Can you work these out from the model? Positions are in its coordinate system, mm. Face numbers are marked on the shaded views. A direction names the side the tool comes from. Give positions to 0.01 mm unless a question says otherwise; leave off trailing zeros. Order: outer loops, then holes, each group sorted by start corner. A loop starts at its lowest first (then second) coordinate and runs counter-clockwise, first axis right, second up.
Item 1: I want a section at D-D, the plane x = 25. Write out the boundary of the cut face in (y, z), then the cut area to 3 significant figures.
Item 2: If I drill on line 1 along X through (y, z) = (-4.25, -3.88); line 2 along Z through (x, y) = (25, -4.5); line 3 along Y through (x, z) = (10, 1.15), over which ranges is the centre line in solid material (lowest first)?
Item 3: I want a section at B-B, the plane y = -8. Write out the boundary of the cut face in (x, z), then the cut area to 3 significant figures.
Item 4: If we mould it in two halves opening along Z, with no side actions, what happens to the marked faces 1, 2 and 3? For each: +Z half, -Z half, draft (parallel to the pull), parting line (faces both ways), or undercut.
Item 5: I want a section at C-C, the plane z = -3.88. Write out the boundary of the cut face in (x, y), then the cut area to 3 significant figures.
Item 6: Which directions (+Z, -Z, +X, -X, +Y, -Y) give clear straight access to the entire face, cutting with the end or side of a thin tool? Please do the marked faces 4 and 5.
Item 7: I want a section at A-A, the plane x = 12. Write out the boundary of the cut face in (y, z).
Item 8: I'm going to push flat-ended pins straight in: pin 1 Ø1 at (y, z) = (-14, -4) entering from -X; pin 2 Ø2.5 at (x, z) = (24, -3) entering from +Y; pin 3 Ø3 at (x, y) = (10, -8) entering from -Z; pin 4 Ø1 at (x, y) = (3.5, -5.5) entering from -Z. Where does each tip first touch, or does it pass through?
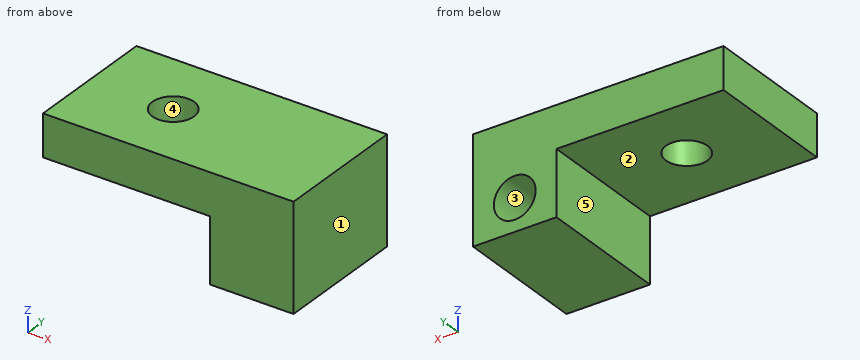
Autodesk Inventor part; units mm, degrees
ref_plane "YZ Plane" through (0, 0, 0) normal (1, 0, 0) x (0, 1, 0)
ref_plane "XZ Plane" through (0, 0, 0) normal (0, 1, 0) x (-1, 0, 0)
ref_plane "XY Plane" through (0, 0, 0) normal (0, 0, 1) x (1, 0, 0)
sketch "Sketch1" plane through (0, 0, 0) normal (0, 0, 1) x (1, 0, 0)
  line L0 (0, 0) -> (20, 0)
  line L1 (20, 0) -> (20, -16)
  line L2 (20, -16) -> (0, -16)
  line L3 (0, -16) -> (0, 0)
  circle A0 centre (10, -8) radius 2.5
  dimension "d0" = 20
  dimension "d1" = 16
  dimension "d2" = 8
  dimension "d3" = 10
  dimension "d4" = 5
extrude "Extrusion1" add sketch "Sketch1" along normal blind 5
sketch "Sketch2" plane through (0, 0, 0) normal (0, 1, 0) x (1, 0, 0)
  line L0 (20, 0) -> (20, -5)
  line L1 (20, 0) -> (30, 0)
  line L2 (30, 0) -> (30, 7.76)
  line L3 (30, 7.76) -> (20, 7.76)
  line L4 (20, 7.76) -> (20, 0)
  line L5 (20, -5) -> (30, -5)
  line L6 (30, -5) -> (30, 0)
  line L7 (30, 0) -> (20, 0)
  line L8 (20, 0) -> (20, -5)
  circle A0 centre (25, 3.88) radius 2.5
  point P0 (0, 0)
  dimension "d7" = 10
  dimension "d8" = 7.76
  dimension "d9" = 5
extrude "Extrusion2" add sketch "Sketch2" against normal blind 16
sketch "Sketch3" plane through (0, -16, 0) normal (0, -1, 0) x (1, 0, 0)
  line L0 (30, -7.76) -> (30, 5)
  line L1 (0, 0) -> (20, 0)
  line L2 (30, -7.76) -> (20, -7.76)
  line L3 (20, -7.76) -> (20, 0)
  line L4 (20, 0) -> (30, 0)
  line L5 (30, 0) -> (30, -7.76)
extrude "Extrusion3" add sketch "Sketch3" against normal blind 9
properties part number "cover mount L v01"
Results list:
1. outline: (-16, -7.76) - (0, -7.76) - (0, -6.38) - (-7, -6.38) - (-7, -1.38) - (0, -1.38) - (0, 5) - (-16, 5) - close
1. area: 169 mm2
2. line 1: x = 20 to 22.5, 27.5 to 30
2. line 2: z = -7.76 to -6.38, -1.38 to 5
2. line 3: y = -16 to -10.5, -5.5 to 0
3. outline: (0, 0) - (7.5, 0) - (7.5, 5) - (0, 5) - close; (12.5, 0) - (20, 0) - (20, -7.76) - (30, -7.76) - (30, 5) - (12.5, 5) - close
3. area: 203 mm2
4. face 1: draft
4. face 2: -Z half
4. face 3: undercut
5. outline: (20, -16) - (30, -16) - (30, 0) - (27.5, 0) - (27.5, -7) - (22.5, -7) - (22.5, 0) - (20, 0) - close
5. area: 125 mm2
6. face 4: +Z, -Z
6. face 5: -Z, -X, +Y, -Y
7. outline: (-16, 0) - (-9.5, 0) - (-9.5, 5) - (-16, 5) - close; (-6.5, 0) - (0, 0) - (0, 5) - (-6.5, 5) - close
8. pin 1: stops at x = 20
8. pin 2: stops at y = 0
8. pin 3: passes through
8. pin 4: stops at z = 0
